Part model, mm, in its own coordinate system. Face numbers are marked on the shaded views. Give positions to 0.01 mm unless a question says otherwise; leave off trailing zeros. Order: outer loops, then holes, each group sorted by start corner. A loop starts at its lowest first (then second) coordinate and runs counter-clockwise, first axis right, second up. Notation, with made-up numbers: (24, 30) -> (50, 30) arc R37 ccw to (50, 68) -> close; hole circle Ø2 at (2.25, -22). An arc over 180 degrees is marked (long way). Write item = value, one per line. Start each with the question number.
(1) Saw through at B-B, the plane y = 0. List the corners of the cut face in (x, z).
(2) Saw through at A-A, the plane z = 54. List the corners of the cut face in (x, y), then the cut area to 3 significant figures.
(3) Flat gauge pins, fed straight in: pin 1 (8 mm diameter, centred on x = 3.5, y = -1, fed in from +Z); pin 2 (8 mm diameter, centred on y = -15, z = 21.5, fed in from -X); pin 3 (3 mm diameter, centred on x = 18, y = -8.5, fed in from -Z); pin 4 (6 mm diameter, centred on x = 19, y = 10.5, fed in from -Z). Where does each tip first touch, or does it go through?
(4) Saw through at C-C, the plane x = 11.5. List the corners of the cut face in (y, z), then the cut area to 3 significant figures.
(5) Two-plate mould, pull along Y, no slides. Class the marked faces 1 and 2: pulls with the +Y half, pulls with the -Y half, needs draft (parallel to the pull), parting line crosses it, or undercut.
(6) Saw through at D-D, the plane y = -9. List the corners of the cut face in (x, z), then the cut area to 3 significant figures.
(7) Probe line 1 along Y through (x, z) = (0, 11); line 2 along Z through (x, y) = (-4, -15.5). List the from-to ranges inside material, lowest first. Write a range as from..to.
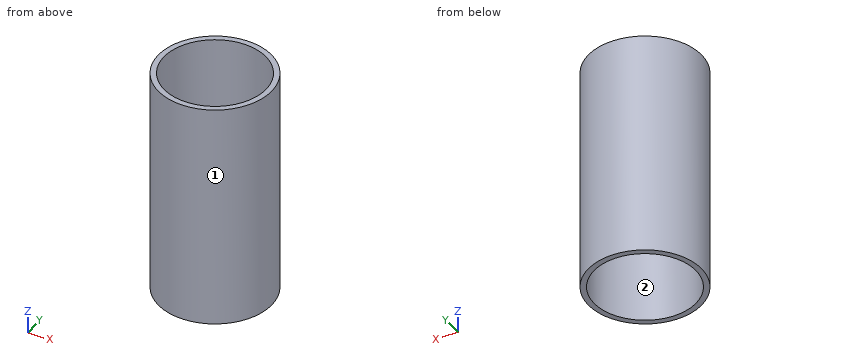
from build123d import *

# Parameters (mm, degrees)
F0_R     = 25.4
F1_DEPTH = 101.6
F2_R     = 22.86
F3_DEPTH = 44.45
F4_R     = 22.86
F5_DEPTH = 44.45
F7_DEPTH = 57.151


with BuildPart() as f1:
    # F0 (on Top) → F1 (new body)
    with BuildSketch(Plane.XY):
        Circle(F0_R)
    extrude(amount=F1_DEPTH)

    # F2 (on face) → F3 (cut)
    with BuildSketch(Plane(origin=(0, 0, 0), x_dir=(1, 0, 0), z_dir=(0, 0, -1))):
        Circle(F2_R)
    extrude(amount=-F3_DEPTH, mode=Mode.SUBTRACT)

    # F4 (on face) → F5 (cut)
    with BuildSketch(Plane.XY.offset(101.6)):
        Circle(F4_R)
    extrude(amount=-F5_DEPTH, mode=Mode.SUBTRACT)

    # F6 (on face) → F7 (cut, through all)
    with BuildSketch(Plane.XY.offset(57.15)):
        Polygon((6.35, 3.666174), (0, 7.332348), (-6.35, 3.666174), (-6.35, -3.666174), (0, -7.332348), (6.35, -3.666174), align=None)
    extrude(amount=-F7_DEPTH, mode=Mode.SUBTRACT)


solid = f1.part
Results list:
q1.outline = (-25.4, 0) -> (-22.86, 0) -> (-22.86, 44.45) -> (-6.35, 44.45) -> (-6.35, 57.15) -> (-22.86, 57.15) -> (-22.86, 101.6) -> (-25.4, 101.6) -> close; (6.35, 44.45) -> (22.86, 44.45) -> (22.86, 0) -> (25.4, 0) -> (25.4, 101.6) -> (22.86, 101.6) -> (22.86, 57.15) -> (6.35, 57.15) -> close
q2.outline = circle Ø50.8 at (0, 0); hole (-6.35, -3.67) -> (0, -7.33) -> (6.35, -3.67) -> (6.35, 3.67) -> (0, 7.33) -> (-6.35, 3.67) -> close
q2.area = 1,890 mm^2
q3.pin_1 = 57.15
q3.pin_2 = -22.89
q3.pin_3 = 44.45
q3.pin_4 = 0
q4.outline = (-22.65, 0) -> (-19.76, 0) -> (-19.76, 44.45) -> (19.76, 44.45) -> (19.76, 0) -> (22.65, 0) -> (22.65, 101.6) -> (19.76, 101.6) -> (19.76, 57.15) -> (-19.76, 57.15) -> (-19.76, 101.6) -> (-22.65, 101.6) -> close
q4.area = 1,090 mm^2
q5.face_1 = parting line crosses it
q5.face_2 = undercut
q6.outline = (-23.75, 0) -> (-21.01, 0) -> (-21.01, 44.45) -> (21.01, 44.45) -> (21.01, 0) -> (23.75, 0) -> (23.75, 101.6) -> (21.01, 101.6) -> (21.01, 57.15) -> (-21.01, 57.15) -> (-21.01, 101.6) -> (-23.75, 101.6) -> close
q6.area = 1,090 mm^2
q7.line_1 = -25.4..-22.86, 22.86..25.4
q7.line_2 = 44.45..57.15
